Design review of the part built by this model. Coordinates are the model's own, in mm. Face numbers are marked on the shaded views. Round coordinates to 2 decimals unless told otherwise and drop trailing zeros.
from build123d import *

# Parameters (mm, degrees)
SKETCH1_W           = 90
SKETCH1_H           = 40
BOSS_EXTRUDE1_DEPTH = 30
FILLET1_R           = 3
FILLET2_R           = 3


with BuildPart() as part:
    # Sketch1 → Boss-Extrude1 (new body)
    with BuildSketch(Plane(origin=(0, 0, 0), x_dir=(1, 0, 0), z_dir=(0, 1, 0))):
        with Locations((45, 20)):
            Rectangle(SKETCH1_W, SKETCH1_H)
    extrude(amount=BOSS_EXTRUDE1_DEPTH)

    # Fillet1
    fillet1_edges = [part.edges().sort_by_distance(p)[0] for p in [
        (45, 30, 0),
    ]]
    fillet(fillet1_edges, radius=FILLET1_R)

    # Fillet2
    fillet2_edges = [part.edges().sort_by_distance(p)[0] for p in [
        (45, 30, -40),
    ]]
    fillet(fillet2_edges, radius=FILLET2_R)


solid = part.part
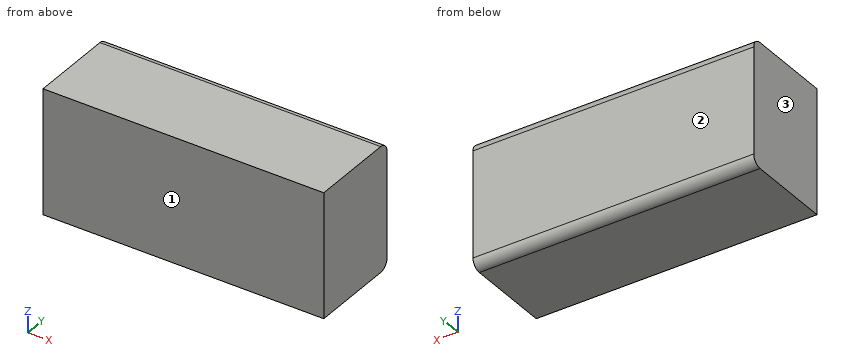
1) To check wall thickness, follow line 1 along Z through (x, y) = (36.5, 27.25); line 2 along Z through (x, y) = (79, 28.75). State the ranges of each line that lie inside material, in increasing order.
Results:
line 1: z = -39.99 to -0.01
line 2: z = -39.44 to -0.56
2) The part is to be moulded in two halves that separate along Y. For the marked faces 1, 2 and 3, say which applies: released by +Y, released by -Y, zero draft, split by the parting line, or undercut.
Results:
face 1: released by -Y
face 2: released by +Y
face 3: zero draft
3) Clearance check with a flat-ended pin moving along its axis: P1, Ø1, axis at x = 62.5, z = -9.5, coming from the -Y side. State where the tip first meets the part, or that it passes through.
Results:
P1: stops at y = 0
